Autodesk Inventor part; units mm, degrees
ref_plane "YZ Plane" through (0, 0, 0) normal (1, 0, 0) x (0, 1, 0)
ref_plane "XZ Plane" through (0, 0, 0) normal (0, 1, 0) x (-1, 0, 0)
ref_plane "XY Plane" through (0, 0, 0) normal (0, 0, 1) x (1, 0, 0)
sketch "Sketch2" plane through (0, 0, 0) normal (1, 0, 0) x (0, 1, 0)
  line L0 (-138.9896, 11.158) -> (0, 11.158)
  line L1 (-139.8126, 0.9719) -> (-139.8126, 10.1861)
  line L2 (0, 0) -> (-138.9896, 0)
  line L3 (0, 11.158) -> (0, 0)
  circle A0 centre (-122.5, 5.579) radius 1.5
  circle A1 centre (-70, 5.579) radius 1.5
  circle A2 centre (-17.5, 5.579) radius 1.5
  line L4 (-138.9896, 0) -> (-139.8126, 0)
  line L5 (-139.8126, 0) -> (-139.8126, 0.9719)
  line L6 (-138.9896, 11.158) -> (-139.8126, 11.158)
  line L7 (-139.8126, 11.158) -> (-139.8126, 10.1861)
extrude "Extrusion2" add sketch "Sketch2" along normal blind 2
properties part number "tutup_fin_fix"
CAD build for the part. Positions are in the model's coordinates, mm. Give positions to 0.01 mm unless a question says otherwise; leave off trailing zeros. Write each loop counter-clockwise with the first axis right and the second up, starting at its lowest first coordinate (ties: lowest second). Pieces come first, ordered by that corner, then holes. Notation, with made-up numbers: M 3.25,-22.5 L 17.25,-22.5 A24 ccw 17.25,14.5 Z; hole C -12.75,28.25 d3. An arc over 180 degrees is marked long. Put each result on its own line as item: value. Start each with the question number.
(1) Mould opens along Z. For faces 1 (the face through (0, -71, 7)), 2 (the face through (0.99, -19, 5.51)) say: +Z half, -Z half, draft (parallel to the pull), parting line (faces both ways), or undercut.
(2) Probe L1, parallel to Y at x = 0.3, z = 6.5; L2, parallel to Z at x = 0.8, y = -17.5; L3, parallel to Y at x = 0.3, z = 6.75. List the from-to ranges inside material, lowest first.
(3) Band-saw the part on A-A, the plane y = -122.5. Write the cut outline in (x, z).
Response values:
1. face 1: draft
1. face 2: undercut
2. L1: y = -139.81 to -123.68, -121.32 to -71.18, -68.82 to -18.68, -16.32 to 0
2. L2: z = 0 to 4.08, 7.08 to 11.16
2. L3: y = -139.81 to -123.44, -121.56 to -70.94, -69.06 to -18.44, -16.56 to 0
3. outline: M 0,0 L 2,0 L 2,4.08 L 0,4.08 Z; M 0,7.08 L 2,7.08 L 2,11.16 L 0,11.16 Z
